from build123d import *

# Parameters (mm, degrees)
SKETCH2_W           = 127
SKETCH2_H           = 124.46
BOSS_EXTRUDE1_DEPTH = 12.7
FILLET1_R           = 2.54
SKETCH3_W           = 115.38555028
SKETCH3_H           = 6.35
SKETCH3_W_2         = 43.18
SKETCH3_H_2         = 10.16
CUT_EXTRUDE1_DEPTH  = 12.7


with BuildPart() as part:
    # Sketch2 → Boss-Extrude1 (new body)
    with BuildSketch(Plane(origin=(0, 0, 0), x_dir=(1, 0, 0), z_dir=(0, 1, 0))):
        with Locations((0, 19.05)):
            Rectangle(SKETCH2_W, SKETCH2_H)
    extrude(amount=BOSS_EXTRUDE1_DEPTH)

    # Fillet1
    fillet1_edges = [part.edges().sort_by_distance(p)[0] for p in [
        (0, 12.7, 43.18),
        (63.5, 12.7, -19.05),
        (0, 12.7, -81.28),
        (-63.5, 12.7, -19.05),
    ]]
    fillet(fillet1_edges, radius=FILLET1_R)

    # Sketch3 → Cut-Extrude1 (cut)
    with BuildSketch(Plane(origin=(0, 12.7, 0), x_dir=(1, 0, 0), z_dir=(0, 1, 0))):
        with Locations((-2.54e-06, 62.865)):
            Rectangle(SKETCH3_W, SKETCH3_H)
        with Locations((0, -33.02)):
            Rectangle(SKETCH3_W_2, SKETCH3_H_2)
        with Locations((-2.54e-06, -1.905)):
            Rectangle(SKETCH3_W, SKETCH3_H)
    extrude(amount=-CUT_EXTRUDE1_DEPTH, mode=Mode.SUBTRACT)


solid = part.part
Can you work these out from the model? Positions are in its coordinate system, mm. A direction names the side the tool comes from. Round coordinates to 2 decimals unless told otherwise and drop trailing zeros. Loops run counter-clockwise (first coordinate to the right, second up) from the corner with the lowest first, then second, coordinate; pieces in that order, holes last. Notation, with made-up numbers: (-5, 48.5) - (47, 48.5) arc R22 ccw to (47, 55.5) - close; hole circle Ø9 at (-28, -16). An arc over 180 degrees is marked (long way). Write item = value, one per line. Start each with the question number.
(1) If we section it at B-B (z = 2): Please give me the cut outline in (x, y), and give its area (3 significant figures).
(2) If I drill on probe 1 along Z at (x, y) = (1.5, 2); probe 2 along Z at (x, y) = (-41, 4.25); probe 3 along X at (y, z) = (3, 34), over which ranges is the centre line in solid material (lowest first)? Write a range as [from, to].
(3) For P1, Ø3, axis at x = -24.5, z = -44.5, coming from the -Y side, with a flat end and sliding along its axis, tell me the tip position at first contact or that it passes through.
(4) If we section it at C-C (y = 4): Please give me the cut outline in (x, z), and give its area (3 significant figures).
(5) For faces 5 (the face through (0, 6, 27.94)), 6 (the face through (-1, 5, 43.18)), which set-ups out of +Z, -Z, +X, -X, +Y, -Y let a thin tool reach every point of the face, with its end or its side?
(6) If we mould it in two halves opening along X, with no side actions, what happens to faces 1 (the face through (-1, 6, -59.69)), 2 (the face through (-1, 0, -20)), 3 (the face through (-63.5, 5, -18)), 4 (the face through (63.5, 5, -18))? For each: released by +X, released by -X, zero draft, split by the parting line, or undercut.
(7) If we section it at A-A (x = -27): Please give me the cut outline in (y, z), and give its area (3 significant figures).
Ans:
q1.outline = (-63.5, 0) - (-57.69, 0) - (-57.69, 12.7) - (-60.96, 12.7) arc R2.54 ccw to (-63.5, 10.16) - close; (57.69, 0) - (63.5, 0) - (63.5, 10.16) arc R2.54 ccw to (60.96, 12.7) - (57.69, 12.7) - close
q1.area = 145 mm²
q2.probe_1 = [-81.28, -66.04], [-59.69, -1.27], [5.08, 27.94], [38.1, 43.18]
q2.probe_2 = [-81.28, -66.04], [-59.69, -1.27], [5.08, 43.18]
q2.probe_3 = [-63.5, -21.59], [21.59, 63.5]
q3.P1 = 0
q4.outline = (-63.5, -81.28) - (63.5, -81.28) - (63.5, 43.18) - (-63.5, 43.18) - close; hole (-57.69, -66.04) - (57.69, -66.04) - (57.69, -59.69) - (-57.69, -59.69) - close; hole (-57.69, -1.27) - (57.69, -1.27) - (57.69, 5.08) - (-57.69, 5.08) - close; hole (-21.59, 27.94) - (21.59, 27.94) - (21.59, 38.1) - (-21.59, 38.1) - close
q4.area = 13,900 mm²
q5.face_5 = +Y, -Y
q5.face_6 = +Z, +X, -X, +Y, -Y
q6.face_1 = undercut
q6.face_2 = zero draft
q6.face_3 = released by -X
q6.face_4 = released by +X
q7.outline = (0, -81.28) - (10.16, -81.28) arc R2.54 ccw to (12.7, -78.74) - (12.7, -66.04) - (0, -66.04) - close; (0, -59.69) - (12.7, -59.69) - (12.7, -1.27) - (0, -1.27) - close; (0, 5.08) - (12.7, 5.08) - (12.7, 40.64) arc R2.54 ccw to (10.16, 43.18) - (0, 43.18) - close
q7.area = 1,420 mm²
